```python
from build123d import *

# Parameters (mm, degrees)
BOSS_EXTRUDE1_DEPTH = 6
SKETCH2_R           = 5
CUT_EXTRUDE1_DEPTH  = 6
SKETCH11_R          = 4.999999998
CUT_EXTRUDE2_DEPTH  = 10
SKETCH12_R          = 5
SKETCH12_R_2        = 2.5
CUT_EXTRUDE3_DEPTH  = 10
CUT_EXTRUDE4_DEPTH  = 10
CUT_EXTRUDE5_DEPTH  = 10
BOSS_EXTRUDE2_START = -6
SKETCH14_R          = 2.5
BOSS_EXTRUDE2_DEPTH = 6
SKETCH14_3_R        = 2.5
CUT_EXTRUDE6_DEPTH  = 6


with BuildPart() as part:
    # Sketch1 → Boss-Extrude1 (new body)
    with BuildSketch(Plane.XY):
        Polygon((-82.808015356, -91.768584182), (61.688025962, -107.113154668), (120.9333121, 25.569013955), (13.052871288, 122.915674351), (-112.866193993, 50.397050544), align=None)
    extrude(amount=BOSS_EXTRUDE1_DEPTH)

    # Sketch2 → Cut-Extrude1 (cut)
    with BuildSketch(Plane.XY.offset(6)):
        Circle(SKETCH2_R)
    extrude(amount=-CUT_EXTRUDE1_DEPTH, mode=Mode.SUBTRACT)

    # Sketch11 → Cut-Extrude2 (cut)
    with BuildSketch(Plane.XY.offset(6)):
        with Locations((-6.54719671, -61.653339044)):
            Circle(SKETCH11_R)
        with Locations((-4.672797652, -44.002584721)):
            Circle(SKETCH11_R)
        with Locations((-2.798398593, -26.351830398)):
            Circle(SKETCH11_R)
        with Locations((-8.975995491, -84.524739011)):
            Circle(SKETCH11_R)
    cut_extrude2 = extrude(amount=-CUT_EXTRUDE2_DEPTH, mode=Mode.SUBTRACT)

    # Sketch12 → Cut-Extrude3 (cut)
    with BuildSketch(Plane.XY.offset(6)):
        with Locations((48.851207931, -21.813057641)):
            Circle(SKETCH12_R)
        with Locations((25.110433983, -11.212319348)):
            Circle(SKETCH12_R)
        with Locations((84.822429951, -20.352343286)):
            Circle(SKETCH12_R_2)
        with Locations((72.591981879, -32.413795933)):
            Circle(SKETCH12_R)
    cut_extrude3 = extrude(amount=-CUT_EXTRUDE3_DEPTH, mode=Mode.SUBTRACT)

    # Sketch11_3 → Cut-Extrude4 (cut)
    with BuildSketch(Plane.XY.offset(6)):
        Polygon((8.29449613, -101.443097727), (8.875295839, -95.973849909), (23.791426251, -97.557849113), (23.210626543, -103.027096932), align=None)
        Polygon((-29.414485521, -97.438641123), (-28.833685813, -91.969393305), (-43.749816225, -90.3853941), (-44.330615934, -95.854641919), align=None)
    cut_extrude4 = extrude(amount=-CUT_EXTRUDE4_DEPTH, mode=Mode.SUBTRACT)

    # Mirror3: Cut-Extrude2 across plane
    add(cut_extrude2.mirror(Plane(origin=(0, 0, 0), x_dir=(0, 0, 1), z_dir=(-0.4077207035645653, -0.9131066903077734, 0))), mode=Mode.SUBTRACT)

    # Mirror4: Cut-Extrude3 across plane
    add(cut_extrude3.mirror(Plane(origin=(0, 0, 0), x_dir=(0, 0, 1), z_dir=(0.742423441529948, -0.6699309169360882, 0))), mode=Mode.SUBTRACT)

    # Mirror5: Cut-Extrude2 across plane
    add(cut_extrude2.mirror(Plane(origin=(0, 0, 0), x_dir=(0, 0, 1), z_dir=(0.742423441529948, -0.6699309169360882, 0))), mode=Mode.SUBTRACT)

    # Mirror6: Cut-Extrude4 across plane
    add(cut_extrude4.mirror(Plane(origin=(0, 0, 0), x_dir=(0, 0, 1), z_dir=(-0.4077207035645653, -0.9131066903077734, 0))), mode=Mode.SUBTRACT)

    # Mirror7: Cut-Extrude4 across plane
    add(cut_extrude4.mirror(Plane(origin=(0, 0, 0), x_dir=(0, 0, 1), z_dir=(0.742423441529948, -0.6699309169360882, 0))), mode=Mode.SUBTRACT)

    # Sketch13 → Cut-Extrude5 (cut)
    with BuildSketch(Plane.XY.offset(6)):
        Polygon((79.910592339, -66.30299436), (102.710745723, -15.241146353), (97.688658926, -12.998682483), (74.888505542, -64.060530491), align=None)
    cut_extrude5 = extrude(amount=-CUT_EXTRUDE5_DEPTH, mode=Mode.SUBTRACT)

    # Mirror8: Cut-Extrude5 across plane
    add(cut_extrude5.mirror(Plane(origin=(0, 0, 0), x_dir=(0, 0, 1), z_dir=(0.742423441529948, -0.6699309169360882, 0))), mode=Mode.SUBTRACT)

    # Sketch14 → Boss-Extrude2 (add)
    with BuildSketch(Plane(origin=(0, 0, 0), x_dir=(-1, 0, 0), z_dir=(0, 0, -1)).offset(BOSS_EXTRUDE2_START)):
        with Locations((-84.822429951, -20.352343286)):
            Circle(SKETCH14_R)
    extrude(amount=BOSS_EXTRUDE2_DEPTH)

    # Sketch14_3 → Cut-Extrude6 (cut)
    with BuildSketch(Plane(origin=(0, 0, 0), x_dir=(-1, 0, 0), z_dir=(0, 0, -1))):
        with Locations(Location((-71.775367437, -49.571757376, 0), (0, 0, 180))):
            Circle(SKETCH14_3_R)
    extrude(amount=-CUT_EXTRUDE6_DEPTH, mode=Mode.SUBTRACT)


solid = part.part
```
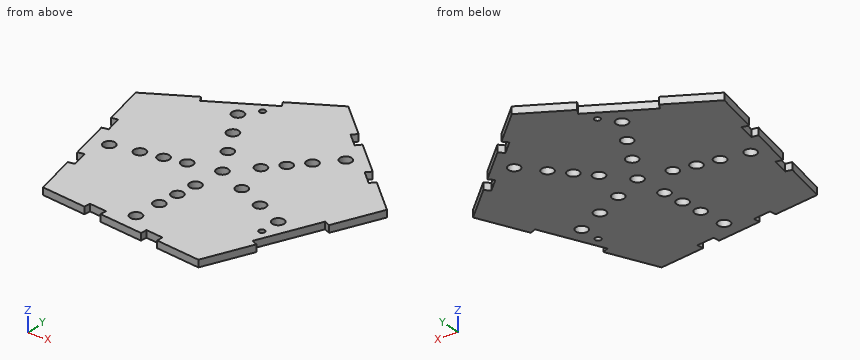
Here's how the part is built. I have some questions about the finished solid (model axes, mm). Give positions to 0.01 mm unless a question says otherwise; leave off trailing zeros. Answer as a JSON object with one key per item and string values. Group by question number.
Item 1: Please list where these lines run through material, in increasing order: probe 1 along Y at (x, z) = (21.5, 1) (3 decimals); probe 2 along Y at (x, z) = (20.5, 4); probe 3 along X at (y, z) = (-7, 2).
Item 2: For P1, Ø6.5, axis at x = -28.93, y = 82.29, coming from the -Z side, with a flat end and sliding along its axis, tell me the tip position at first contact or that it passes through.
Item 3: If we section it at A-A on z = 3.25: Give the number of separate pieces and of enclosed holes in the cut face, and give its area (3 significant figures).
Result set:
{
 "1": {"probe 1": "-97.315 to -14.671, -7.753 to 16.363, 22.985 to 115.293", "probe 2": "-97.21 to -13.15, -9.28 to 15.5, 23.85 to 116.2", "probe 3": "-100.73 to -47.81, -38.78 to -30.69, -21.16 to 22.42, 27.8 to 106.39"},
 "2": {"P1": "z = 0"},
 "3": {"separate pieces": "1", "enclosed holes": "21", "area": "33,700 mm²"}
}
